```python
from build123d import *

# Parameters (mm, degrees)
ESQUISSE1_W             = 78.786961771
ESQUISSE1_H             = 77.107895372
BOSS_EXTRU_1_DEPTH      = 90
ESQUISSE3_W             = 55.543823951
ESQUISSE3_H             = 42.068648109
BOSS_EXTRU_3_DEPTH      = 50
ESQUISSE4_W             = 18.786498619
ESQUISSE4_H             = 27.73494317
ESQUISSE4_W_2           = 31.884127938
ESQUISSE4_H_2           = 30.645527463
ESQUISSE4_W_3           = 18.521900048
ESQUISSE4_H_3           = 13.494527178
ESQUISSE4_W_4           = 27.253652927
ENL_V_MAT_EXTRU_1_DEPTH = 110


with BuildPart() as part:
    # Esquisse1 → Boss.-Extru.1 (new body)
    with BuildSketch(Plane(origin=(0, 0, 0), x_dir=(1, 0, 0), z_dir=(0, 1, 0))):
        with Locations((39.393480886, 38.553947686)):
            Rectangle(ESQUISSE1_W, ESQUISSE1_H)
    extrude(amount=BOSS_EXTRU_1_DEPTH)

    # Esquisse3 → Boss.-Extru.3 (add)
    with BuildSketch(Plane(origin=(78.786961771, 0, 0), x_dir=(0, 0, -1), z_dir=(1, 0, 0))):
        with Locations((49.335983396, 21.034324055)):
            Rectangle(ESQUISSE3_W, ESQUISSE3_H)
    extrude(amount=BOSS_EXTRU_3_DEPTH)

    # Esquisse4 → Enlèv. mat.-Extru.1 (cut)
    with BuildSketch(Plane.XY):
        with Locations((39.78581368, 13.867471585)):
            Rectangle(ESQUISSE4_W, ESQUISSE4_H)
        with Locations((104.28171563, 15.322763732)):
            Rectangle(ESQUISSE4_W_2, ESQUISSE4_H_2)
        with Locations((21.131614346, 67.557028272)):
            Rectangle(ESQUISSE4_W_3, ESQUISSE4_H_3)
        with Locations((57.513918011, 67.557028272)):
            Rectangle(ESQUISSE4_W_4, ESQUISSE4_H_3)
    extrude(amount=-ENL_V_MAT_EXTRU_1_DEPTH, mode=Mode.SUBTRACT)


solid = part.part
```
Check sheet for the modelled part. Datum: model origin and axes. Units: mm. A direction names the side the tool comes from. Give positions to 0.01 mm unless a question says otherwise; leave off trailing zeros. Loops run counter-clockwise (first coordinate to the right, second up) from the corner with the lowest first, then second, coordinate; pieces in that order, holes last. Notation, with made-up numbers: (69.5, -17) - (82.5, -17) arc R25 ccw to (82.5, 17) - close; hole circle Ø4 at (1.5, -19). An arc over 180 degrees is marked (long way). One line per question, with ' | ' between items. Start each with the question number.
1. Cross-section at A-A, the plane z = -4.5. Enter the section's corners in (x, y), plus the area to 3 significant figures.
2. Gauge pin test, flat end, axial feed: pin 1 Ø11 at (y, z) = (71, -51) entering from +X. Record the tip position at first contact, or that the pin passes through.
3. Cross-section at D-D, the plane y = 70. Enter the section's corners in (x, z), plus the area to 3 significant figures.
4. Material ranges on line 1 along X through (y, z) = (20.5, -51); line 2 along X through (y, z) = (61, -24.5); line 3 along X through (y, z) = (9, -12), recorded low to high. Write a range as [from, to].
5. Set-up check for faces 1 (the flat face through (30.393, 14, -38)), 2 (the flat face through (0, 44, -38)), 3 (the flat face through (71.141, 67, -38)): record each of +Z, -Z, +X, -X, +Y, -Y from which the full face is reachable in a straight line by a thin tool's end or side.
6. Draft check along Y on faces 4 (the flat face through (30.393, 67, -38)), 5 (the flat face through (68, 0, -38)), 6 (the flat face through (49.179, 14, -38)). Enter one of: released by +Y, released by -Y, zero draft, split by the parting line, or undercut.
7. Cross-section at C-C, the plane x = 61.5. Enter the section's corners in (y, z), plus the area to 3 significant figures.
8. Cross-section at B-B, the plane y = 9. Enter the section's corners in (x, z), plus the area to 3 significant figures.
Check result:
1) outline: (0, 0) - (30.39, 0) - (30.39, 27.73) - (49.18, 27.73) - (49.18, 0) - (78.79, 0) - (78.79, 90) - (0, 90) - close; hole (11.87, 60.81) - (30.39, 60.81) - (30.39, 74.3) - (11.87, 74.3) - close; hole (43.89, 60.81) - (71.14, 60.81) - (71.14, 74.3) - (43.89, 74.3) - close | area: 5,950 mm2
2) pin 1: stops at x = 78.79
3) outline: (0, -77.11) - (11.87, -77.11) - (11.87, 0) - (0, 0) - close; (30.39, -77.11) - (43.89, -77.11) - (43.89, 0) - (30.39, 0) - close; (71.14, -77.11) - (78.79, -77.11) - (78.79, 0) - (71.14, 0) - close | area: 2,550 mm2
4) line 1: x = [0, 30.39], [49.18, 88.34], [120.22, 128.79] | line 2: x = [0, 11.87], [30.39, 43.89], [71.14, 78.79] | line 3: x = [0, 30.39], [49.18, 78.79]
5) face 1: +Z, -Z, -Y | face 2: +Z, -Z, -X, +Y, -Y | face 3: +Z, -Z
6) face 4: undercut | face 5: released by -Y | face 6: zero draft
7) outline: (0, -77.11) - (60.81, -77.11) - (60.81, 0) - (0, 0) - close; (74.3, -77.11) - (90, -77.11) - (90, 0) - (74.3, 0) - close | area: 5,900 mm2
8) outline: (0, -77.11) - (30.39, -77.11) - (30.39, 0) - (0, 0) - close; (49.18, -77.11) - (88.34, -77.11) - (88.34, -21.56) - (78.79, -21.56) - (78.79, 0) - (49.18, 0) - close; (120.22, -77.11) - (128.79, -77.11) - (128.79, -21.56) - (120.22, -21.56) - close | area: 5,630 mm2
